```python
from build123d import *

# Parameters (mm, degrees)
F1_DEPTH    = 7
F2_T1_DEPTH = 54.3718610795


# Not quite as in the source:
# - a fillet or chamfer that OpenCascade refuses, or shapes differently, is made with other operations: its cross-section is extruded or revolved along the edge and cut away or added


with BuildPart() as f1:
    # F0 (on Top) → F1 (new body)
    with BuildSketch(Plane.XY):
        with BuildLine():
            Line((-25, -4), (25, -4))
            ThreePointArc((25, -4), (29, 0), (25, 4))
            Line((25, 4), (-25, 4))
            ThreePointArc((-25, 4), (-29, 0), (-25, -4))
        make_face()
    extrude(amount=F1_DEPTH)

    # F2: chamfer of 0.5 on 4 edges, made by hand

    # F2_s2 → F2_t1 (cut)
    with BuildSketch(Plane.YZ.offset(-27.1859305398)):
        Polygon((-4, 6.5), (-3.5, 7), (-4, 7), align=None)
        Polygon((4, 6.5), (3.5, 7), (4, 7), align=None)
        Polygon((-4, 0.5), (-3.5, 0), (-4, 0), align=None)
        Polygon((4, 0.5), (3.5, 0), (4, 0), align=None)
    extrude(amount=F2_T1_DEPTH, mode=Mode.SUBTRACT)


solid = f1.part
```
Could you check a few things on this model? Use its own coordinates, in mm. Round coordinates to 2 decimals unless told otherwise and drop trailing zeros. Write each loop counter-clockwise with the first axis right and the second up, starting at its lowest first coordinate (ties: lowest second). Pieces come first, ordered by that corner, then holes. Notation, with made-up numbers: M 49.5,49.5 L 88.5,49.5 A21 cw 88.5,84.5 Z; hole C -6.5,47 d1. An arc over 180 degrees is marked long. Write each question's results on one line, items separated by ' | '. Start each with the question number.
1. Imagine slicing it at A-A on z = 1. List the corners of the cut face in (x, y) for me.
2. I'm going to push flat-ended pins straight in: pin 1 Ø4 at (y, z) = (-2.5, 1.5) entering from +X; pin 2 Ø1.5 at (y, z) = (-3, 6) entering from +X. Where does each tip first touch, or does it pass through?
3. I need wall thicknesses on L1, parallel to X at y = 0.25, z = 1.5; L2, parallel to X at y = 3, z = 6.75; L3, parallel to Y at x = 25.5, z = 4.5. Which ranges of each line are inside material? Lowest first, please. Write a range as from..to.
4. Imagine slicing it at B-B on y = 3. List the corners of the cut face in (x, z) for me, and give its area (3 significant figures).
Result sheet:
1) outline: M -25,-4 L 25,-4 A4 ccw 25,4 L -25,4 A4 ccw Z
2) pin 1: stops at x = 28.97 | pin 2: stops at x = 28.31
3) L1: x = -28.99..28.99 | L2: x = -27.65..27.65 | L3: y = -3.97..3.97
4) outline: M -27.65,0 L 27.65,0 L 27.65,7 L -27.65,7 Z | area: 387 mm^2
